Input: part model. Units: mm. Frame: model coordinates. Face numbers are marked on the shaded views. A direction names the side the tool comes from. Coordinates: 2 decimals unless noted, no trailing zeros. Loops run counter-clockwise (first coordinate to the right, second up) from the corner with the lowest first, then second, coordinate; pieces in that order, holes last.
(1) Contact query for a flat-ended pin moving along its axis: P1, Ø24, axis at x = -7.5, y = 4, coming from the +Z side. Output: stop coordinate, or through.
(2) Section A-A, the plane y = -21. Return loops of the section in (x, z).
(3) Line query: L1, parallel to X at y = 2.5, z = 29; L2, parallel to Y at x = 28, z = 30.5; L3, parallel to Z at x = 37, y = -6. Output: solid intervals per line, ascending.
(4) Section B-B, the plane z = 7. Return loops of the section in (x, y).
(5) Section D-D, the plane x = -2. Return loops of the section in (y, z).
(6) Mould query, pull axis Y, two halves, no side actions, for the marked faces 1, 2 and 3. Classes: released by +Y, released by -Y, zero draft, split by the parting line, or undercut.
(7) Section C-C, the plane x = 29.5. Return loops of the section in (y, z), then the cut area to 4 significant figures.
(8) Set-up query: the marked faces 4 and 5. Return all of +Z, -Z, +X, -X, +Y, -Y with unobstructed straight access to the full face (end or side cutting, diameter ignored); none if empty.
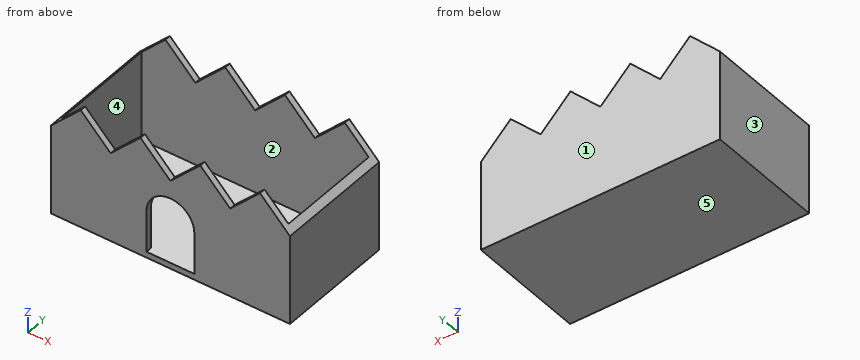
```python
from build123d import *

# Parameters (mm, degrees)
F0_W     = 100
F0_H     = 50
F1_DEPTH = 50
F3_DEPTH = 50
F4_T     = -2.5
F6_DEPTH = 2.5


with BuildPart() as f1:
    # F0 (on Top) → F1 (new body)
    with BuildSketch(Plane.XY):
        Rectangle(F0_W, F0_H)
    extrude(amount=F1_DEPTH)

    # F2 (on face) → F3 (cut, through all)
    with BuildSketch(Plane.XZ.offset(25)):
        Polygon((-50, 50), (-50, 37.5), (-37.5, 50), align=None)
        Polygon((-12.5, 50), (-37.5, 50), (-25, 37.5), align=None)
        Polygon((12.5, 50), (-12.5, 50), (0, 37.5), align=None)
        Polygon((37.5, 50), (12.5, 50), (25, 37.5), align=None)
        Polygon((37.5, 50), (50, 37.5), (50, 50), align=None)
    extrude(amount=-F3_DEPTH, mode=Mode.SUBTRACT)

    # F4
    f4_openings = [f1.faces().sort_by_distance(p)[0] for p in [
        (-31.25, 0, 43.75),
        (-6.25, 0, 43.75),
        (18.75, 0, 43.75),
        (43.75, 0, 43.75),
        (31.25, 0, 43.75),
        (6.25, 0, 43.75),
        (-18.75, 0, 43.75),
        (-43.75, 0, 43.75),
    ]]
    offset(amount=F4_T, openings=f4_openings)

    # F5 (on face) → F6 (cut, through all)
    with BuildSketch(Plane.XZ.offset(25)):
        with BuildLine():
            ThreePointArc((-10, 20), (0, 10), (10, 20))
            Line((10, 20), (-10, 20))
        make_face()
        with BuildLine():
            Line((-10, 20), (10, 20))
            ThreePointArc((10, 20), (0, 30), (-10, 20))
        make_face()
        with BuildLine():
            Line((10, 2.5), (10, 20))
            ThreePointArc((10, 20), (0, 10), (-10, 20))
            Line((-10, 20), (-10, 2.5))
            Line((-10, 2.5), (10, 2.5))
        make_face()
    extrude(amount=-F6_DEPTH, mode=Mode.SUBTRACT)


solid = f1.part
```
Report:
1. P1: stops at z = 2.5
2. outline: (-50, 0) - (50, 0) - (50, 37.5) - (47.5, 40) - (47.5, 2.5) - (-47.5, 2.5) - (-47.5, 40) - (-50, 37.5) - close
3. L1: x = -50 to -47.5, 47.5 to 50
3. L2: y = -25 to -22.5, 22.5 to 25
3. L3: z = 0 to 2.5
4. outline: (-50, -25) - (-10, -25) - (-10, -22.5) - (-47.5, -22.5) - (-47.5, 22.5) - (47.5, 22.5) - (47.5, -22.5) - (10, -22.5) - (10, -25) - (50, -25) - (50, 25) - (-50, 25) - close
5. outline: (-25, 0) - (25, 0) - (25, 39.5) - (22.5, 39.5) - (22.5, 2.5) - (-25, 2.5) - close; (-25, 29.8) - (-22.5, 29.8) - (-22.5, 39.5) - (-25, 39.5) - close
6. face 1: released by +Y
6. face 2: undercut
6. face 3: zero draft
7. outline: (-25, 0) - (25, 0) - (25, 42) - (22.5, 42) - (22.5, 2.5) - (-22.5, 2.5) - (-22.5, 42) - (-25, 42) - close
7. area: 322.5 mm2
8. face 4: +Z
8. face 5: -Z, +X, -X, +Y, -Y
